Check sheet for the modelled part. Datum: model origin and axes. Units: mm. A direction names the side the tool comes from. Coordinates: 2 decimals unless noted, no trailing zeros. One line per item, written item: value. Start each with the question number.
1) Gauge pin test, flat ends, axial feed: P1, Ø3, axis at x = 27, y = -11.5, coming from the -Z side; P2, Ø1, axis at y = -12, z = 19.5, coming from the -X side; P3, Ø15.5, axis at x = 17, z = 21, coming from the +Y side; P4, Ø12, axis at x = 7.5, z = 18, coming from the -Y side. Record the tip position at first contact, or that the pin passes through.
2) Scan lines: line 1 along X through (y, z) = (1, 13.5); line 2 along Y through (x, z) = (7.5, 12.5); line 3 along Y through (x, z) = (3, 23). Record each from-to range of solid material in increasing order. Write a range as [from, to].
3) Set-up check for faces 4 (the flat face through (35, 0, 13)), 5 (the flat face through (17, 2.4, 16)): record each of +Z, -Z, +X, -X, +Y, -Y from which the full face is reachable in a straight line by a thin tool's end or side.
4) Draft check along X on faces 1 (the flat face through (2, 0, 16)), 2 (the flat face through (17, 4, 0)), 3 (the flat face through (0, 0, 13)). Enter one of: +X half, -X half, draft (parallel to the pull), parting line (faces both ways), or undercut.
```python
from build123d import *

# Parameters (mm, degrees)
F4_DEPTH = 35
F6_DEPTH = 33
F7_R     = 4


# Not quite as in the source:
# - a feature names something its author has since deleted; it is built from what else it names


with BuildPart() as f4:
    # F3 (on Right) → F4 (new body)
    with BuildSketch(Plane.YZ):
        with BuildLine():
            Line((-20, 0), (0, 0))
            Line((0, 0), (0, 37))
            add(Edge.make_bspline(
                [(0, 37), (-8.5256332532, 37.0518802553), (-17.6288448274, 20.054070279), (-20, 0)],
                knots=[0.5, 0.5, 0.5, 0.5, 1, 1, 1, 1], degree=3))
        make_face()
        with BuildLine():
            Line((0, 37), (0, 0))
            Line((0, 0), (20, 0))
            add(Edge.make_bspline(
                [(20, 0), (16.4736881852, 19.8465492576), (8.5256332532, 36.9481197447), (0, 37)],
                knots=[0, 0, 0, 0, 0.5, 0.5, 0.5, 0.5], degree=3))
        make_face()
    extrude(amount=F4_DEPTH)

    # F5 (on face) → F6 (cut)
    with BuildSketch(Plane(origin=(0, 0, 0), x_dir=(1, 0, 0), z_dir=(0, 0, -1))):
        Polygon((2, 2.4), (2, 0), (2, -2.4), (33, -2.4), (33, 0), (33, 2.4), align=None)
    extrude(amount=-F6_DEPTH, mode=Mode.SUBTRACT)

    # F7
    f7_edges = [f4.edges().sort_by_distance(p)[0] for p in [
        (35, -0.138558, 36.999345),
        (0, -0.138558, 36.999345),
    ]]
    fillet(f7_edges, radius=F7_R)


solid = f4.part
```
Answers:
1. P1: stops at z = 0
1. P2: stops at x = 0.02
1. P3: stops at y = 16.86
1. P4: stops at y = -17.71
2. line 1: x = [0, 2], [33, 35]
2. line 2: y = [-17.57, -2.4], [2.4, 17.09]
2. line 3: y = [-13.68, -2.4], [2.4, 13.14]
3. face 4: +Z, -Z, +X, +Y, -Y
3. face 5: -Z
4. face 1: undercut
4. face 2: draft
4. face 3: -X half
